Verification items for the finished model (mm, model axes). A direction names the side the tool comes from. Coordinates: 2 decimals unless noted, no trailing zeros. Order: outer loops, then holes, each group sorted by start corner. A loop starts at its lowest first (then second) coordinate and runs counter-clockwise, first axis right, second up. Notation, with made-up numbers: (12, 51) -> (32, 51) arc R15 ccw to (32, 60) -> close; hole circle Ø5 at (15, 70.5). An arc over 180 degrees is marked (long way). Answer as CSV lines item,"result".
```python
from build123d import *

# Parameters (mm, degrees)
F0_R     = 3.75
F0_R_2   = 1.7
F1_DEPTH = 3.8
F3_DEPTH = 2.5


# Not quite as in the source:
# - a feature of the source that left no trace in its solid (it failed there, or was rolled back) is left out


with BuildPart() as f1:
    # F0 (on Top) → F1 (new body)
    with BuildSketch(Plane.XY):
        with Locations((56.9799989462, -33.0372825265)):
            Circle(F0_R)
        with Locations((56.9799989462, -33.0372825265)):
            Circle(F0_R_2, mode=Mode.SUBTRACT)
    extrude(amount=F1_DEPTH)

    # F2 (on face) → F3 (cut)
    with BuildSketch(Plane(origin=(0, 0, 0), x_dir=(1, 0, 0), z_dir=(0, 0, -1))):
        Polygon((59.9799989462, 31.3052317189), (59.9799989462, 34.7693333341), (56.9799989462, 36.5013841416), (53.9799989462, 34.7693333341), (53.9799989462, 31.3052317189), (56.9799989462, 29.5731809114), align=None)
    extrude(amount=-F3_DEPTH, mode=Mode.SUBTRACT)


solid = f1.part
```
Item 1: Section check A-A, the plane y = -33.5. Record the boundary of the cut face in (x, z).
Answer list:
outline,"(53.26, 0) -> (53.98, 0) -> (53.98, 2.5) -> (55.34, 2.5) -> (55.34, 3.8) -> (53.26, 3.8) -> close; (58.62, 2.5) -> (59.98, 2.5) -> (59.98, 0) -> (60.7, 0) -> (60.7, 3.8) -> (58.62, 3.8) -> close"
Item 2: Section check B-B, the plane x = 58. Record the boundary of the cut face in (y, z).
Answer list:
outline,"(-36.65, 0) -> (-35.91, 0) -> (-35.91, 2.5) -> (-34.4, 2.5) -> (-34.4, 3.8) -> (-36.65, 3.8) -> close; (-31.68, 2.5) -> (-30.16, 2.5) -> (-30.16, 0) -> (-29.43, 0) -> (-29.43, 3.8) -> (-31.68, 3.8) -> close"
Item 3: Section check C-C, the plane z = 0.4. Record the boundary of the cut face in (x, y), plus the area to 3 significant figures.
Answer list:
outline,"circle Ø7.5 at (56.98, -33.04); hole (53.98, -34.77) -> (56.98, -36.5) -> (59.98, -34.77) -> (59.98, -31.31) -> (56.98, -29.57) -> (53.98, -31.31) -> close"
area,"13.0 mm2"
Item 4: Release check for a two-part mould opening along Y. For faces 1 (the flat face through (58, -35, 3.8)), 2 (the cylindrical face through (56.49, -29.32, 1.87)), 3 (the flat face through (55.46, -30.45, 1.23)) record: +Y half, -Y half, draft (parallel to the pull), parting line (faces both ways), or undercut.
Answer list:
face 1,"draft"
face 2,"parting line"
face 3,"undercut"
Item 5: Section check D-D, the plane x = 54.25. Record the boundary of the cut face in (y, z).
Answer list:
outline,"(-35.61, 0) -> (-34.93, 0) -> (-34.93, 2.5) -> (-31.15, 2.5) -> (-31.15, 0) -> (-30.47, 0) -> (-30.47, 3.8) -> (-35.61, 3.8) -> close"
Item 6: Depth check by flat-ended pin: pin 1 Ø1.8 at (x, y) = (56, -33.5) entering from -Z. Enter the tip coordinate at first touch or a pass-through.
Answer list:
pin 1,"z = 2.5"
Item 7: Tool access check on faces 4 (the flat face through (53.98, -33, 1)), 5 (the cylindrical face through (58.55, -33.69, 3.14)). Record the directions out of +Z, -Z, +X, -X, +Y, -Y that give a thin tool (end or side, any length) a straight path to the whole face; none if there is none.
Answer list:
face 4,"-Z"
face 5,"+Z, -Z"
Item 8: Thickness scan on line 1 (Z direction, x = 55.75, y = -35.25); line 2 (X direction, y = -31.5, z = 1.9); line 3 (Y direction, x = 58.25, z = 3.6). Record the ranges inside material, lowest first.
Answer list:
line 1,"2.5 to 3.8"
line 2,"53.56 to 53.98, 59.98 to 60.4"
line 3,"-36.57 to -34.17, -31.91 to -29.51"
